Can you work these out from the model? Positions are in its coordinate system, mm. Face numbers are marked on the shaded views. A direction names the side the tool comes from. Round coordinates to 2 decimals unless told otherwise and drop trailing zeros. Loops run counter-clockwise (first coordinate to the right, second up) from the corner with the lowest first, then second, coordinate; pieces in that order, holes last.
(1) Will these pins go through, and if not, where does the flat tip stop? pin 1 Ø12 at (y, z) = (2, 47) entering from +X; pin 2 Ø8 at (y, z) = (2, 13.5) entering from -X; pin 3 Ø8 at (y, z) = (8.5, 35) entering from -X.
(2) If I drill on line 1 along Y through (x, z) = (-7.25, 9); line 2 along X through (y, z) = (-8.5, 6); line 3 along Y through (x, z) = (-1.25, 64.5), over which ranges is the centre line in solid material (lowest first)?
(3) I want a section at C-C on z = 65. Write out the boundary of the cut face in (x, y), plus the area to 3 significant figures.
(4) I want a section at A-A on x = 0. Write out the boundary of the cut face in (y, z), plus the area to 3 significant figures.
(5) I want a section at D-D on z = 24. Write out the boundary of the cut face in (x, y), plus the area to 3 significant figures.
(6) Which directions (+Z, -Z, +X, -X, +Y, -Y) give clear straight access to the entire face, cutting with the end or side of a thin tool? Please do the marked faces 1 and 2.
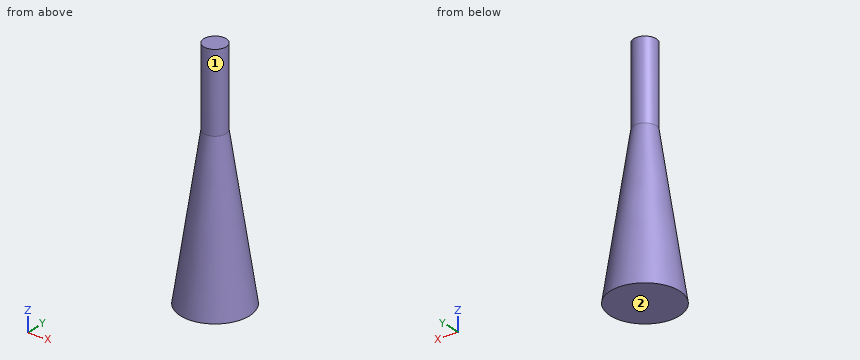
from build123d import *

# Parameters (mm, degrees)
F2_W      = 56.300126
F2_H      = 25.4
F3_DEPTH  = 10.16
F3_FACE_R = 3.643881
F4_DEPTH  = 25.4


with BuildPart() as f1:
    # F0 (on Front) → F1 (revolve)
    with BuildSketch(Plane.XZ):
        Polygon((0, 75.375971), (0, 0), (11.176, 0), align=None)
    revolve(axis=Axis((0, 0, 32.428367), (0, 0, -1)))

    # F2 (on Right) → F3 (cut, symmetric)
    with BuildSketch(Plane.YZ):
        with Locations((-3.274256, 63.5)):
            Rectangle(F2_W, F2_H)
    extrude(amount=F3_DEPTH, both=True, mode=Mode.SUBTRACT)

    # F3_face (on face) → F4 (join)
    with BuildSketch(Plane.XY.offset(50.8)):
        Circle(F3_FACE_R)
    extrude(amount=F4_DEPTH)


solid = f1.part
Filled sheet:
1. pin 1: stops at x = 5.05
1. pin 2: stops at x = -9.71
1. pin 3: stops at x = -4.04
2. line 1: y = -6.66 to 6.66
2. line 2: x = -5.79 to 5.79
2. line 3: y = -3.42 to 3.42
3. outline: circle Ø7.29 at (0, 0)
3. area: 41.7 mm2
4. outline: (-11.18, 0) - (11.18, 0) - (3.64, 50.8) - (3.64, 76.2) - (-3.64, 76.2) - (-3.64, 50.8) - close
4. area: 938 mm2
5. outline: circle Ø15.24 at (0, 0)
5. area: 182 mm2
6. face 1: +Z
6. face 2: -Z, +X, -X, +Y, -Y
